The listing builds one solid part. Answer for the finished solid, in the listing's coordinates (mm). A direction names the side the tool comes from. Coordinates: 2 decimals unless noted, no trailing zeros. Loops run counter-clockwise (first coordinate to the right, second up) from the corner with the lowest first, then second, coordinate; pieces in that order, holes last. Notation, with made-up numbers: (60, 51) - (94, 51) arc R21 ccw to (94, 77) - close; hole circle Ø3 at (-6.5, 53.25). An arc over 180 degrees is marked (long way). Use one line per item in the form item = value. Start each with the question number.
```python
from build123d import *

# Parameters (mm, degrees)
SKETCH1_R            = 304.8
BOSS_EXTRUDE1_DEPTH  = 28.575
SKETCH2_W            = 50.8
SKETCH2_H            = 50.8
BOSS_EXTRUDE2_DEPTH  = 63.5
SKETCH3_R            = 304.8
BOSS_EXTRUDE3_DEPTH  = 225.425
BOSS_EXTRUDE8_DEPTH  = 88.9
SKETCH10_R           = 304.8
BOSS_EXTRUDE11_DEPTH = 6.35
SKETCH11_R           = 304.8
SKETCH11_R_2         = 302.26
BOSS_EXTRUDE12_DEPTH = 12.7
BOSS_EXTRUDE10_REACH = 537.362
SKETCH9_R            = 304.81653601
SKETCH9_R_2          = 298.178711987
SKETCH12_R           = 31.75
SKETCH12_R_2         = 19.05
BOSS_EXTRUDE13_DEPTH = 0.254
CIRPATTERN1_COUNT    = 5


with BuildPart() as part:
    # Sketch1 → Boss-Extrude1 (new body)
    with BuildSketch(Plane(origin=(0, 0, 0), x_dir=(1, 0, 0), z_dir=(0, 1, 0))):
        with Locations(Location((0, 0, 0), (0, 0, 270))):
            Circle(SKETCH1_R)
    extrude(amount=BOSS_EXTRUDE1_DEPTH)

    # Sketch2 → Boss-Extrude2 (add)
    with BuildSketch(Plane(origin=(0, 28.575, 0), x_dir=(1, 0, 0), z_dir=(0, 1, 0))):
        Polygon((245.765281759, 171.222045256), (201.771191247, 145.822045256), (227.171191247, 101.827954744), (271.165281759, 127.227954744), align=None)
        with Locations((0, 273.05)):
            Rectangle(SKETCH2_W, SKETCH2_H)
        Polygon((271.165281759, -127.227954744), (227.171191247, -101.827954744), (201.771191247, -145.822045256), (245.765281759, -171.222045256), align=None)
        with Locations((0, -273.05)):
            Rectangle(SKETCH2_W, SKETCH2_H)
        Polygon((-245.765281759, -171.222045256), (-201.771191247, -145.822045256), (-227.171191247, -101.827954744), (-271.165281759, -127.227954744), align=None)
        Polygon((-271.165281759, 127.227954744), (-227.171191247, 101.827954744), (-201.771191247, 145.822045256), (-245.765281759, 171.222045256), align=None)
    extrude(amount=BOSS_EXTRUDE2_DEPTH)

    # Sketch3 → Boss-Extrude3 (add)
    with BuildSketch(Plane(origin=(0, 92.075, 0), x_dir=(1, 0, 0), z_dir=(0, 1, 0))):
        with Locations(Location((0, 0, 0), (0, 0, 270))):
            Circle(SKETCH3_R)
    extrude(amount=BOSS_EXTRUDE3_DEPTH)

    # Sketch6 → Boss-Extrude8 (add)
    with BuildSketch(Plane(origin=(0, 317.5, 0), x_dir=(1, 0, 0), z_dir=(0, 1, 0))):
        Polygon((94.292689271, 94.292689271), (302.26, 1.27), (302.26, -1.27), (94.292689271, -94.292689271), (1.27, -302.26), (-1.27, -302.26), (-94.292689271, -94.292689271), (-302.26, -1.27), (-302.26, 1.27), (-94.292689271, 94.292689271), (-1.27, 302.26), (1.27, 302.26), align=None)
    extrude(amount=BOSS_EXTRUDE8_DEPTH)

    # Sketch10 → Boss-Extrude11 (add)
    with BuildSketch(Plane(origin=(0, 406.4, 0), x_dir=(1, 0, 0), z_dir=(0, 1, 0))):
        with Locations(Location((0, 0, 0), (0, 0, 270))):
            Circle(SKETCH10_R)
    extrude(amount=BOSS_EXTRUDE11_DEPTH)

    # Sketch11 → Boss-Extrude12 (add)
    with BuildSketch(Plane(origin=(0, 317.5, 0), x_dir=(1, 0, 0), z_dir=(0, 1, 0))):
        with Locations(Location((0, 0, 0), (0, 0, 270))):
            Circle(SKETCH11_R)
        Circle(SKETCH11_R_2, mode=Mode.SUBTRACT)
    extrude(amount=BOSS_EXTRUDE12_DEPTH)

    # Boss-Extrude10: up to this face of the body (flat: up to its plane)
    boss_extrude10_end = Plane(part.part.faces().sort_by_distance((0, 0, 0))[0])
    # Sketch9 → Boss-Extrude10 (add, up to the picked face)
    with BuildSketch(Plane(origin=(0, 317.5, 0), x_dir=(1, 0, 0), z_dir=(0, 1, 0)), mode=Mode.PRIVATE) as boss_extrude10_sk1:
        with Locations(Location((0, 0, 0), (0, 0, 270))):
            Circle(SKETCH9_R)
        Circle(SKETCH9_R_2, mode=Mode.SUBTRACT)
    boss_extrude10_tool1 = split(extrude(boss_extrude10_sk1.sketch, amount=-BOSS_EXTRUDE10_REACH, mode=Mode.PRIVATE), bisect_by=boss_extrude10_end, keep=Keep.BOTH, mode=Mode.PRIVATE)
    add(boss_extrude10_tool1.solids().sort_by(Axis((0, 317.5, -303.954385), (0, -1, 0)))[0])

    # Sketch12 → Boss-Extrude13 (add)
    with BuildSketch(Plane(origin=(0, 412.75, 0), x_dir=(1, 0, 0), z_dir=(0, 1, 0))):
        with Locations(Location((0, -254, 0), (0, 0, 270))):
            Circle(SKETCH12_R)
        with Locations(Location((103.311107341, -232.040546241, 0), (0, 0, 270))):
            Circle(SKETCH12_R_2)
        with Locations(Location((188.758785671, -169.959174015, 0), (0, 0, 270))):
            Circle(SKETCH12_R_2)
    boss_extrude13 = extrude(amount=BOSS_EXTRUDE13_DEPTH)

    # CirPattern1: Boss-Extrude13 ×5 about axis
    cirpattern1_axis = Axis((0, 0, 0), (0, 1, 0))
    for i in range(1, CIRPATTERN1_COUNT):
        add(boss_extrude13.rotate(cirpattern1_axis, i * 360 / CIRPATTERN1_COUNT))


solid = part.part
```
(1) Determine the mould class of faces 3 (the face through (-185.466, 323.761, -241.879)), 4 (the face through (149, 413.004, -205)), 5 (the face through (147.5, 60.77, 259.14)) for opening direction X: +X half, -X half, draft (parallel to the pull), parting line (faces both ways), or undercut.
(2) A cutting plane is placed at C-C (y = 257). Determine the outline of the cut face in (x, z).
(3) Find the intervals of material crossed by probe 1 along Y at (x, z) = (-138.5, -253) (3 decimals); probe 2 along Y at (x, z) = (-117.5, 43.5) (3 decimals); probe 3 along X at (y, z) = (40.5, 167.5), in increasing order. Write a range as from..to.
(4) A cutting plane is placed at D-D (x = 150.5). Determine the outline of the cut face in (y, z) (3 decimals).
(5) For faces 1 (the face through (-253, 413.004, -26)), 2 (the face through (-214.649, 59.88, -123.517)), determine the directions among +Z, -Z, +X, -X, +Y, -Y from which every point of the face is accessible in a straight line to the end or side of a thin tool.
(6) Each of these flat-tipped pins is pushed along its axis until it touches: pin 1 Ø12 at (x, y) = (-89.5, 125.5) entering from +Z; pin 2 Ø4 at (x, y) = (32, 257.5) entering from -Z; pin 3 Ø1.3 at (x, y) = (0, 381) entering from +Z. Where does it stop, or does it pass through?
Evaluation:
q1.face_3 = parting line
q1.face_4 = draft
q1.face_5 = undercut
q2.outline = circle Ø609.63 at (0, 0)
q3.probe_1 = 0..28.575, 92.075..317.5, 406.4..412.75
q3.probe_2 = 0..28.575, 92.075..412.75
q3.probe_3 = -254.67..-239.32, 239.32..254.67
q4.outline = (0, -265.071) - (317.5, -265.071) - (317.5, -265.052) - (330.2, -265.052) - (330.2, -262.128) - (317.5, -262.128) - (317.5, -69.151) - (406.4, -69.151) - (406.4, -265.052) - (412.75, -265.052) - (412.75, -237.218) - (413.004, -237.218) - (413.004, -173.763) - (412.75, -173.763) - (412.75, 265.052) - (406.4, 265.052) - (406.4, 69.151) - (317.5, 69.151) - (317.5, 262.128) - (330.2, 262.128) - (330.2, 265.052) - (317.5, 265.052) - (317.5, 265.071) - (0, 265.071) - close; hole (28.575, -257.411) - (92.075, -257.411) - (92.075, 257.411) - (28.575, 257.411) - close
q5.face_1 = +Z, -Z, +X, -X, +Y
q5.face_2 = none
q6.pin_1 = 293.16
q6.pin_2 = -303.34
q6.pin_3 = 302.26
